```python
from build123d import *

# Parameters (mm, degrees)
SKETCH5_R           = 1.5
BOSS_EXTRUDE1_DEPTH = 3.5
SKETCH6_W           = 18
SKETCH6_H           = 10
SKETCH6_R           = 1.25
BOSS_EXTRUDE2_DEPTH = 3.5
FILLET1_R           = 2
FILLET2_R           = 0.2


with BuildPart() as part:
    # Sketch5 → Boss-Extrude1 (new body)
    with BuildSketch(Plane.XY):
        with BuildLine():
            Line((52.244364221, 93.802541786), (-62.755635779, 93.802541786))
            Line((-62.755635779, 93.802541786), (-62.755635779, 83.802541786))
            Line((-62.755635779, 83.802541786), (-54.423503372, 70))
            Line((-54.423503372, 70), (-10.03072393, 70))
            Line((-10.03072393, 70), (-10.03072393, 60))
            ThreePointArc((-10.03072393, 60), (-6.03072393, 56), (-2.03072393, 60))
            Line((-2.03072393, 60), (-2.03072393, 70))
            Line((-2.03072393, 70), (38.111411694, 70))
            Line((38.111411694, 70), (52.244364221, 83.802541786))
            Line((52.244364221, 83.802541786), (52.244364221, 93.802541786))
        make_face()
        with Locations((-6.03072393, 60)):
            Circle(SKETCH5_R, mode=Mode.SUBTRACT)
        with BuildLine():
            Line((16.46927607, 89.802541786), (-28.53072393, 89.802541786))
            ThreePointArc((-28.53072393, 89.802541786), (-33.03072393, 85.302541786), (-28.53072393, 80.802541786))
            Line((-28.53072393, 80.802541786), (16.46927607, 80.802541786))
            ThreePointArc((16.46927607, 80.802541786), (20.96927607, 85.302541786), (16.46927607, 89.802541786))
        make_face(mode=Mode.SUBTRACT)
    extrude(amount=BOSS_EXTRUDE1_DEPTH)

    # Sketch6 → Boss-Extrude2 (add)
    # profile 1 of 2: a face of its own
    with BuildSketch(Plane(origin=(0, 93.802541786, 0), x_dir=(1, 0, 0), z_dir=(0, 1, 0))):
        with Locations((-53.755635779, 5)):
            Rectangle(SKETCH6_W, SKETCH6_H)
        with Locations(Location((-58.755635779, 5, 0), (0, 0, 180))):
            Circle(SKETCH6_R, mode=Mode.SUBTRACT)
        with Locations(Location((-48.755635779, 5, 0), (0, 0, 180))):
            Circle(SKETCH6_R, mode=Mode.SUBTRACT)
    # profile 2 of 2: a face of its own
    with BuildSketch(Plane(origin=(0, 93.802541786, 0), x_dir=(1, 0, 0), z_dir=(0, 1, 0))):
        with Locations((43.244364221, 5)):
            Rectangle(SKETCH6_W, SKETCH6_H)
        with Locations((38.244364221, 5)):
            Circle(SKETCH6_R, mode=Mode.SUBTRACT)
        with Locations((48.244364221, 5)):
            Circle(SKETCH6_R, mode=Mode.SUBTRACT)
    extrude(amount=-BOSS_EXTRUDE2_DEPTH)

    # Fillet1
    fillet1_edges = [part.edges().sort_by_distance(p)[0] for p in [
        (52.244364221, 83.802541786, 1.75),
        (38.111411694, 70, 1.75),
        (-2.03072393, 70, 1.75),
        (-10.03072393, 70, 1.75),
        (-54.423503372, 70, 1.75),
        (-62.755635779, 83.802541786, 1.75),
    ]]
    fillet(fillet1_edges, radius=FILLET1_R)

    # Fillet2
    fillet2_edges = [part.edges().sort_by_distance(p)[0] for p in [
        (-2.03072393, 64, 0),
        (-6.03072393, 56, 0),
        (-7.53072393, 60, 0),
        (-33.03072393, 85.302541786, 0),
        (-6.03072393, 80.802541786, 0),
        (20.96927607, 85.302541786, 0),
        (-6.03072393, 89.802541786, 0),
        (-62.755635779, 87.330975349, 0),
        (-62.755635779, 90.302541786, -5),
        (-53.755635779, 90.302541786, 0),
        (-44.755635779, 92.052541786, 0),
        (-44.755635779, 93.802541786, -5),
        (-5.255635779, 93.802541786, 0),
        (52.244364221, 90.302541786, -5),
        (43.244364221, 90.302541786, 0),
        (34.244364221, 92.052541786, 0),
        (34.244364221, 93.802541786, -5),
        (-10.03072393, 64, 0),
        (-32.662699153, 70, 0),
        (18.633041615, 70, 0),
        (52.244364221, 87.473700585, 0),
        (45.167974716, 76.891589411, 0),
        (-58.737365074, 77.146100601, 0),
        (-62.682345408, 83.822948285, 0),
        (-54.277728874, 70.258275609, 0),
        (38.051233908, 70.147747242, 0),
        (52.087564977, 83.868579168, 0),
        (-10.616510367, 69.414213562, 0),
        (-1.444937492, 69.414213562, 0),
    ]]
    fillet(fillet2_edges, radius=FILLET2_R)


solid = part.part
```
Geometry check sheet. Reference: the model listing, model coordinates, mm. A direction names the side the tool comes from. Give positions to 0.01 mm unless a question says otherwise; leave off trailing zeros. Order: outer loops, then holes, each group sorted by start corner. A loop starts at its lowest first (then second) coordinate and runs counter-clockwise, first axis right, second up. Notation, with made-up numbers: (-11.75, -28) -> (36.25, -28) arc R9 cw to (36.25, -21) -> close; hole circle Ø3 at (44.25, -29). An arc over 180 degrees is marked (long way). Write each question's results on one line, items separated by ' | '. Start each with the question number.
(1) Scan lines: line 1 (X direction, y = 92, z = -9.5); line 2 (Y direction, x = -53, z = -9); line 3 (Z direction, x = 40, y = 74.5). Record each from-to range of solid material in increasing order.
(2) Sectioned sample at A-A (x = -20.5). Enter the section's corners in (y, z).
(3) Sectioned sample at B-B (z = -2.5). Enter the section's corners in (x, y), plus the area to 3 significant figures.
(4) Mould release check, pull along X, two halves, no side actions. Record for faces 4 (the face through (-6, 79, 3.5)), 5 (the face through (-1.46, 69.4, 1.87)), 6 (the face through (-33.03, 85.4, 1.83)): pulls with the +X half, pulls with the -X half, needs draft (parallel to the pull), parting line crosses it, or undercut.
(5) Gauge pin test, flat ends, axial feed: P1, Ø1.5, axis at x = 25, z = 1.5, coming from the -Y side; P2, Ø2, axis at x = 48.24, z = -5, coming from the -Y side; P3, Ø1, axis at y = 65.5, z = 1.5, coming from the -X side; P4, Ø3, axis at x = -54.5, z = -6, coming from the -Y side. Record the tip position at first contact, or that the pin passes through.
(6) Access from +Z, -Z, +X, -X, +Y, -Y to the whole of each face (thin tool, end or side, straight path). Record for faces 1 (the face through (-6, 80.803, 2)), 2 (the face through (-10.031, 64, 2)), 3 (the face through (-6, 79, 0)).
Answer below:
1) line 1: -62.76 to -44.76, 34.24 to 52.24 | line 2: 90.3 to 93.8 | line 3: 0 to 3.5
2) outline: (70, 0.2) arc R0.2 ccw to (70.2, 0) -> (80.6, 0) arc R0.2 ccw to (80.8, 0.2) -> (80.8, 3.5) -> (70, 3.5) -> close; (89.8, 0.2) arc R0.2 ccw to (90, 0) -> (93.6, 0) arc R0.2 ccw to (93.8, 0.2) -> (93.8, 3.5) -> (89.8, 3.5) -> close
3) outline: (-62.76, 90.5) arc R0.2 ccw to (-62.56, 90.3) -> (-44.76, 90.3) -> (-44.76, 93.6) arc R0.2 ccw to (-44.96, 93.8) -> (-62.76, 93.8) -> close; (34.24, 90.3) -> (52.04, 90.3) arc R0.2 ccw to (52.24, 90.5) -> (52.24, 93.8) -> (34.44, 93.8) arc R0.2 ccw to (34.24, 93.6) -> close | area: 126 mm2
4) face 4: needs draft | face 5: pulls with the +X half | face 6: undercut
5) P1: y = 70 | P2: through | P3: x = -10.03 | P4: y = 90.3
6) face 1: +Z, -Z | face 2: +Z, -Z, -X, -Y | face 3: -Z, -Y
